CAD build for the part. Positions are in the model's coordinates, mm. A direction names the side the tool comes from. Give positions to 0.01 mm unless a question says otherwise; leave off trailing zeros. Write each loop counter-clockwise with the first axis right and the second up, starting at its lowest first coordinate (ties: lowest second). Pieces come first, ordered by that corner, then holes. Notation, with made-up numbers: (9.5, -32.5) -> (40.5, -32.5) arc R19 cw to (40.5, -6.5) -> close; hole circle Ø11 at (14.5, 78). An arc over 180 degrees is marked (long way). Use one line per item in the form item = value. Start each with the question number.
from build123d import *

# Parameters (mm, degrees)
BOSS_EXTRUDE1_DEPTH = 6.35
SKETCH2_R           = 2.286
CUT_EXTRUDE1_DEPTH  = 55.254423783
FILLET1_R           = 1.5875


with BuildPart() as part:
    # Sketch1 → Boss-Extrude1 (new, symmetric)
    with BuildSketch(Plane.XY):
        with BuildLine():
            Line((12.7, -21.997045256), (12.7, -38.1))
            Line((12.7, -38.1), (9.525, -38.1))
            Line((9.525, -38.1), (9.525, -26.940768363))
            ThreePointArc((9.525, -26.940768363), (-14.563355395, 24.585347357), (19.05, -21.298547486))
            Line((19.05, -21.298547486), (19.05, -38.1))
            Line((19.05, -38.1), (15.875, -38.1))
            Line((15.875, -38.1), (15.875, -19.827868645))
            ThreePointArc((15.875, -19.827868645), (-14.328607331, 20.9726253), (12.7, -21.997045256))
        make_face()
    extrude(amount=BOSS_EXTRUDE1_DEPTH, both=True)

    # Sketch2 → Cut-Extrude1 (cut, through all)
    with BuildSketch(Plane.ZY.offset(-9.525)):
        with Locations(Location((0, -33.3375, 0), (0, 0, 270))):
            Circle(SKETCH2_R)
    extrude(amount=-CUT_EXTRUDE1_DEPTH, mode=Mode.SUBTRACT)

    # Fillet1
    fillet1_edges = [part.edges().sort_by_distance(p)[0] for p in [
        (17.4625, -38.1, -6.35),
        (17.4625, -38.1, 6.35),
        (12.7, -21.997045256, 0),
        (9.525, -26.940768363, 0),
        (19.05, -21.298547486, 0),
        (15.875, -19.827868645, 0),
        (11.1125, -38.1, 6.35),
        (11.1125, -38.1, -6.35),
    ]]
    fillet(fillet1_edges, radius=FILLET1_R)


solid = part.part
1) Wall check: line 1 along Y through (x, z) = (0, -3) (3 decimals); line 2 along X through (y, z) = (5, 1.75). Give the ranges that are in metal, low to high. Write a range as from..to.
2) Cut at B-B (x = 18). State how many separate pieces and enclosed holes the cut face has, and give its area (3 significant figures).
3) Cut at D-D (x = -16.5). Give the cut face in (y, z).
4) 3-axis set-ups, long thin cutter, end or side, ignore diameter. For faces 1 (the face through (19.05, -30, 0)), 2 (the face through (9.525, -36, 0)), 3 (the face through (12.7, -30, 0)), 4 (the face through (-14.95, 24.35, 0.09)): which of +Z, -Z, +X, -X, +Y, -Y reach the whole face in a straight line?
5) Two-plate mould, pull along Y, no slides. Class faces 5 (the face through (15.875, -29, 0)), 6 (the face through (11.99, -23.27, 0.09)), 7 (the face through (11.09, -37.62, 5.9)): released by +Y, released by -Y, zero draft, split by the parting line, or undercut.
6) Cut at A-A (y = 0). Give the cut face in (x, z) (3 decimals).
7) Pin check, flat tips, straight feed: pin 1 (5 mm diameter, centred on y = -10.5, z = 1, fed in from -X); pin 2 (3 mm diameter, centred on x = -17.5, z = 5, fed in from +Y); pin 3 (5 mm diameter, centred on x = -17.5, z = 2.5, fed in from +Y). Stop position of each tip, or through.
Final values:
q1.line_1 = -28.575..-25.4, 25.4..28.575
q1.line_2 = -28.13..-24.9, 24.9..28.13
q2.separate_pieces = 2
q2.enclosed_holes = 1
q2.area = 293 mm^2
q3.outline = (-23.33, -6.35) -> (-19.31, -6.35) -> (-19.31, 6.35) -> (-23.33, 6.35) -> close; (19.31, -6.35) -> (23.33, -6.35) -> (23.33, 6.35) -> (19.31, 6.35) -> close
q4.face_1 = +Z, -Z, +X, -Y
q4.face_2 = +Z, -Z, -X, -Y
q4.face_3 = +Z, -Z, -Y
q4.face_4 = +Z, -Z
q5.face_5 = zero draft
q5.face_6 = undercut
q5.face_7 = released by -Y
q6.outline = (-28.575, -6.35) -> (-25.4, -6.35) -> (-25.4, 6.35) -> (-28.575, 6.35) -> close; (25.4, -6.35) -> (28.575, -6.35) -> (28.575, 6.35) -> (25.4, 6.35) -> close
q7.pin_1 = -27.43
q7.pin_2 = 23.68
q7.pin_3 = 24.32
